The listing builds one solid part. Answer for the finished solid, in the listing's coordinates (mm). A direction names the side the tool comes from. Round coordinates to 2 decimals unless told otherwise and drop trailing zeros. Order: outer loops, then holes, each group sorted by start corner. A loop starts at its lowest first (then second) coordinate and runs counter-clockwise, first axis right, second up. Notation, with made-up numbers: (-29, 4) -> (-13, 4) arc R19 cw to (-13, 33) -> close; hole circle Ø4 at (69, 75). An arc over 180 degrees is marked (long way). Return JSON: item names as keys, results as strings. Group by question number.
(1) The part is cut by section C-C (x = 25). Determine the outline of the cut face in (y, z), plus the area to 4 significant figures.
(2) Consider line 1 (Y direction, x = 2, z = -3.69); line 2 (X direction, y = 81, z = -1.5); line 3 (Y direction, x = 53.85, z = -3.69). Determine where each line is inside the solid, lowest interval first. Write a range as [from, to].
(3) The part is cut by section B-B (y = 35). Determine the outline of the cut face in (x, z).
(4) Which of the six approach directions +Z, -Z, +X, -X, +Y, -Y give full straight-line access (tool end or side, diameter ignored) to faces 4 (the face through (53.926, 79.043, -4.107)), 5 (the face through (46.966, 80.667, -4.107)), 6 (the face through (1.5, 96.07, 3.55)), 7 (the face through (11.23, 49, 1.48)), 8 (the face through (2.5, 93, 5))?
(5) Determine the mould class of faces 1 (the face through (53.52, 93, -1)), 2 (the face through (41.2, 81, 2)), 3 (the face through (50, 84, -7.38)) for opening direction Z: +Z half, -Z half, draft (parallel to the pull), parting line (faces both ways), or undercut.
(6) The part is cut by section A-A (z = 6). Count the separate pieces of the cut face and the enclosed holes in it, plus the area to 3 significant figures.
(7) Each of these flat-tipped pins is pushed along its axis until it touches: pin 1 (2.5 mm diameter, centred on y = 25, z = 1, fed in from +X); pin 2 (4.5 mm diameter, centred on y = 3.5, z = 6, fed in from -X); pin 3 (3 mm diameter, centred on y = 91.5, z = -3, fed in from -X); pin 4 (6 mm diameter, centred on x = 23, z = 6.5, fed in from +Y). Where does it stop, or does it pass through?
from build123d import *

# Parameters (mm, degrees)
SKETCH1_W           = 51
SKETCH1_H           = 97.5
BOSS_EXTRUDE2_DEPTH = 3
BOSS_EXTRUDE3_DEPTH = 4
BOSS_EXTRUDE4_DEPTH = 4
SKETCH5_W           = 51
SKETCH5_H           = 1
BOSS_EXTRUDE5_DEPTH = 10
CUT_EXTRUDE1_DEPTH  = 10
FILLET1_R           = 5
SKETCH8_R           = 2.6
BOSS_EXTRUDE6_DEPTH = 7.76
SKETCH9_R           = 3.2
CUT_EXTRUDE2_DEPTH  = 0.8
CUT_EXTRUDE3_START  = -0.8
SKETCH10_R          = 3.2
CUT_EXTRUDE3_DEPTH  = 0.8
FILLET2_R           = 3


with BuildPart() as part:
    # Sketch1 → Boss-Extrude2 (new body)
    with BuildSketch(Plane.XY):
        with Locations((25.5, 48.75)):
            Rectangle(SKETCH1_W, SKETCH1_H)
    extrude(amount=BOSS_EXTRUDE2_DEPTH)

    # Sketch3 → Boss-Extrude3 (add)
    with BuildSketch(Plane.XY.offset(3)):
        Polygon((0, 97.5), (7.5, 97.5), (7.5, 95.5), (2.5, 95.5), (2.5, 90.5), (0, 90.5), align=None)
        Polygon((51, 97.5), (44, 97.5), (44, 95.5), (49, 95.5), (49, 90.5), (51, 90.5), align=None)
        Polygon((51, 0), (44, 0), (44, 2), (49, 2), (49, 7), (51, 7), align=None)
    extrude(amount=BOSS_EXTRUDE3_DEPTH)

    # Sketch4 → Boss-Extrude4 (add)
    with BuildSketch(Plane.XY.offset(3)):
        Polygon((3, 0), (3, 7), (5, 7), (5, 2), (10.869482621, 2), (10.869482621, 0), align=None)
    extrude(amount=BOSS_EXTRUDE4_DEPTH)

    # Sketch5 → Boss-Extrude5 (add)
    with BuildSketch(Plane.XY.offset(3)):
        with Locations((25.5, 60.5)):
            Rectangle(SKETCH5_W, SKETCH5_H)
    extrude(amount=BOSS_EXTRUDE5_DEPTH)

    # Sketch6 → Cut-Extrude1 (cut)
    with BuildSketch(Plane.XY.offset(3)):
        Polygon((39.8, 93.770532131), (9.8, 93.770532131), (9.8, 68.770532131), (41.2, 68.770532131), (41.2, 93.770532131), align=None)
        Polygon((39.8, 50.5), (9.8, 50.5), (9.8, 10.5), (41.2, 10.5), (41.2, 50.5), align=None)
    extrude(amount=-CUT_EXTRUDE1_DEPTH, mode=Mode.SUBTRACT)

    # Fillet1
    fillet1_edges = [part.edges().sort_by_distance(p)[0] for p in [
        (0, 60.5, 13),
        (51, 60.5, 13),
        (9.8, 50.5, 1.5),
        (9.8, 93.770532131, 1.5),
        (41.2, 93.770532131, 1.5),
        (41.2, 10.5, 1.5),
        (9.8, 10.5, 1.5),
        (41.2, 50.5, 1.5),
        (51, 0, 3.5),
        (51, 97.5, 3.5),
        (0, 97.5, 3.5),
        (9.8, 68.770532131, 1.5),
        (41.2, 68.770532131, 1.5),
        (0, 0, 1.5),
    ]]
    fillet(fillet1_edges, radius=FILLET1_R)

    # Sketch8 → Boss-Extrude6 (add)
    with BuildSketch(Plane.ZY):
        Polygon((0, 81.56), (0, 89.53), (0, 92.5), (0, 97.5), (-7.38, 97.5), (-7.38, 70.18), (0, 70.18), align=None)
        with Locations((-3.69, 75.87)):
            Circle(SKETCH8_R, mode=Mode.SUBTRACT)
        with Locations((-3.69, 91.81)):
            Circle(SKETCH8_R, mode=Mode.SUBTRACT)
        with Locations((-3.69, 83.84)):
            Circle(SKETCH8_R, mode=Mode.SUBTRACT)
    boss_extrude6 = extrude(amount=-BOSS_EXTRUDE6_DEPTH)

    # Sketch9 → Cut-Extrude2 (cut)
    with BuildSketch(Plane.ZY):
        with Locations((-3.69, 91.81)):
            Circle(SKETCH9_R)
        with Locations((-3.69, 83.84)):
            Circle(SKETCH9_R)
        with Locations((-3.69, 75.87)):
            Circle(SKETCH9_R)
    cut_extrude2 = extrude(amount=-CUT_EXTRUDE2_DEPTH, mode=Mode.SUBTRACT)

    # Sketch10 → Cut-Extrude3 (cut)
    with BuildSketch(Plane(origin=(7.76, 0, 0), x_dir=(0, 0, -1), z_dir=(1, 0, 0)).offset(CUT_EXTRUDE3_START)):
        with Locations(Location((3.69, 91.81, 0), (0, 0, 180))):
            Circle(SKETCH10_R)
        with Locations(Location((3.69, 83.84, 0), (0, 0, 180))):
            Circle(SKETCH10_R)
        with Locations(Location((3.69, 75.87, 0), (0, 0, 180))):
            Circle(SKETCH10_R)
    cut_extrude3 = extrude(amount=CUT_EXTRUDE3_DEPTH, mode=Mode.SUBTRACT)

    # Mirror2: Boss-Extrude6, Cut-Extrude2, Cut-Extrude3 across plane
    add(boss_extrude6.mirror(Plane(origin=(27.16, 0, 0), x_dir=(0, 0, 1), z_dir=(1, 0, 0))))
    add(cut_extrude2.mirror(Plane(origin=(27.16, 0, 0), x_dir=(0, 0, 1), z_dir=(1, 0, 0))), mode=Mode.SUBTRACT)
    add(cut_extrude3.mirror(Plane(origin=(27.16, 0, 0), x_dir=(0, 0, 1), z_dir=(1, 0, 0))), mode=Mode.SUBTRACT)

    # Fillet2
    fillet2_edges = [part.edges().sort_by_distance(p)[0] for p in [
        (3.88, 97.5, -7.38),
        (3.88, 70.18, -7.38),
        (50.44, 97.5, -7.38),
        (50.44, 70.18, -7.38),
    ]]
    fillet(fillet2_edges, radius=FILLET2_R)


solid = part.part
Answer below:
{
 "1": {"outline": "(0, 0) -> (10.5, 0) -> (10.5, 3) -> (0, 3) -> close; (50.5, 0) -> (68.77, 0) -> (68.77, 3) -> (61, 3) -> (61, 13) -> (60, 13) -> (60, 3) -> (50.5, 3) -> close; (93.77, 0) -> (97.5, 0) -> (97.5, 3) -> (93.77, 3) -> close", "area": "107.5 mm²"},
 "2": {"line 1": "y = [70.18, 73.27], [78.47, 81.24], [86.44, 89.21], [94.41, 97.5]", "line 2": "x = [0, 7.76], [46.56, 54.32]", "line 3": "y = [70.18, 72.67], [79.07, 80.64], [87.04, 88.61], [95.01, 97.5]"},
 "3": {"outline": "(0, 0) -> (9.8, 0) -> (9.8, 3) -> (0, 3) -> close; (41.2, 0) -> (51, 0) -> (51, 3) -> (41.2, 3) -> close"},
 "4": {"face 4": "+X", "face 5": "none", "face 6": "+Z, -X, +Y", "face 7": "+Z, -Z", "face 8": "+Z"},
 "5": {"face 1": "undercut", "face 2": "draft", "face 3": "-Z half"},
 "6": {"separate pieces": "5", "enclosed holes": "0", "area": "136 mm²"},
 "7": {"pin 1": "stops at x = 51", "pin 2": "stops at x = 3", "pin 3": "passes through", "pin 4": "stops at y = 61"}
}
